Model file for the job. Use its own axes, mm. Face numbers are marked on the shaded views. A direction names the side the tool comes from. Coordinates: 2 decimals unless noted, no trailing zeros. Order: outer loops, then holes, each group sorted by start corner. A loop starts at its lowest first (then second) coordinate and runs counter-clockwise, first axis right, second up.
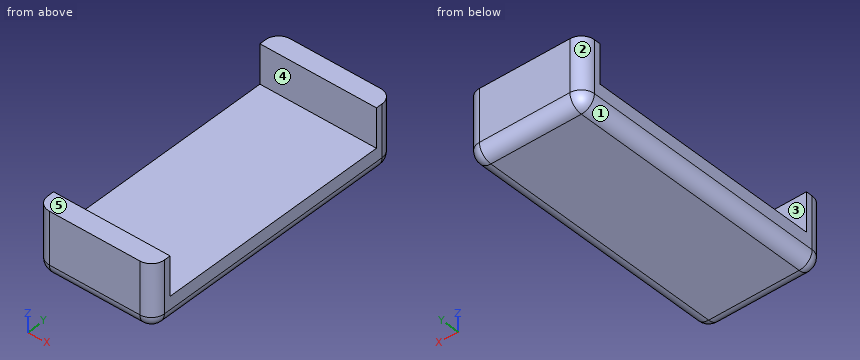
from build123d import *

# Parameters (mm, degrees)
F0_W     = 17.9
F0_H     = 42.2
F1_DEPTH = 4
F2_W     = 17.9
F2_H     = 3
F3_DEPTH = 6
F4_W     = 17.9
F4_H     = 3
F5_DEPTH = 6
F6_R     = 2


with BuildPart() as f1:
    # F0 (on Top) → F1 (new body)
    with BuildSketch(Plane.XY):
        with Locations((-14.323435, -9.50025)):
            Rectangle(F0_W, F0_H)
    extrude(amount=F1_DEPTH)

    # F2 (on face) → F3 (join)
    with BuildSketch(Plane.XY.offset(4)):
        with Locations((-14.323435, 10.09975)):
            Rectangle(F2_W, F2_H)
    extrude(amount=F3_DEPTH)

    # F4 (on face) → F5 (join)
    with BuildSketch(Plane.XY.offset(4)):
        with Locations((-14.323435, -29.10025)):
            Rectangle(F4_W, F4_H)
    extrude(amount=F5_DEPTH)

    # F6
    f6_edges = [f1.edges().sort_by_distance(p)[0] for p in [
        (-23.273435, -9.50025, 0),
        (-5.373435, -9.50025, 0),
        (-14.323435, 11.59975, 0),
        (-14.323435, -30.60025, 0),
        (-5.373435, 11.59975, 5),
        (-23.273435, 11.59975, 5),
        (-5.373435, -30.60025, 5),
        (-23.273435, -30.60025, 5),
    ]]
    fillet(f6_edges, radius=F6_R)


solid = f1.part
Q1. Cut at A-A, the plane z = 6.5. List the corners of the cut face in (x, y).
Established:
outline: (-23.27, -28.6) arc R2 ccw to (-21.27, -30.6) - (-7.37, -30.6) arc R2 ccw to (-5.37, -28.6) - (-5.37, -27.6) - (-23.27, -27.6) - close; (-23.27, 8.6) - (-5.37, 8.6) - (-5.37, 9.6) arc R2 ccw to (-7.37, 11.6) - (-21.27, 11.6) arc R2 ccw to (-23.27, 9.6) - close
Q2. Mould opens along Y. For the marked faces 1, 2 and 3 say: pulls with the +Y half, pulls with the -Y half, needs draft (parallel to the pull), parting line crosses it, or undercut.
Established:
face 1: needs draft
face 2: pulls with the +Y half
face 3: undercut
Q3. Probe line 1 (Y direction, x = -16.5, z = 5.5); line 2 (Z direction, x = -20.25, y = -8); line 3 (Y direction, x = -6.25, z = 7.5). List the from-to ranges inside material, lowest first.
Established:
line 1: y = -30.6 to -27.6, 8.6 to 11.6
line 2: z = 0 to 4
line 3: y = -30.25 to -27.6, 8.6 to 11.25
Q4. Cut at B-B, the plane x = -12.75. List the corners of the cut face in (y, z), plus the area to 3 significant figures.
Established:
outline: (-30.6, 2) arc R2 ccw to (-28.6, 0) - (9.6, 0) arc R2 ccw to (11.6, 2) - (11.6, 10) - (8.6, 10) - (8.6, 4) - (-27.6, 4) - (-27.6, 10) - (-30.6, 10) - close
area: 203 mm2
Q5. Cut at C-C, the plane y = -2. List the corners of the cut face in (x, z).
Established:
outline: (-23.27, 2) arc R2 ccw to (-21.27, 0) - (-7.37, 0) arc R2 ccw to (-5.37, 2) - (-5.37, 4) - (-23.27, 4) - close
Q6. Drop a flat-ended pin along its axis: P1, Ø1, axis at x = -19, y = -14.5, coming from the +Z side. Give the stop position or say it passes through.
Established:
P1: stops at z = 4
Q7. Which spindle directions (+Z, -Z, +X, -X, +Y, -Y) get a long thin tool onto all of the face, cutting with end or side? Do the marked faces 4 and 5. Say none if no direction does.
Established:
face 4: +Z, +X, -X
face 5: +Z, +X, -X, +Y, -Y
Q8. Cut at D-D, the plane x = -22. List the corners of the cut face in (y, z).
Established:
outline: (-30.46, 2) arc R1.86 ccw to (-28.6, 0.14) - (9.6, 0.14) arc R1.86 ccw to (11.46, 2) - (11.46, 10) - (8.6, 10) - (8.6, 4) - (-27.6, 4) - (-27.6, 10) - (-30.46, 10) - close
